Check sheet for the drawn part. Datum: minimum x, y, z corner. Units: mm. Round coordinates to 2 decimals unless told otherwise and drop trailing zeros. Write each loop counter-clockwise with the first axis right and the second up, starting at its lowest first coordinate (ties: lowest second). Pieces come first, ordered by that corner, then holes. Notation, with made-up numbers: (-40, 59) - (-34, 59) arc R13 ccw to (-34, 76) - close; hole circle Ø3 at (4.25, -29.5). An arc over 180 degrees is marked (long way). Answer as a JSON object with one key per item and string values. Group by question number.
1) Section check C-C (z = 4). Enter the section's corners in (x, y).
2) Section check B-B (y = 4). Enter the section's corners in (x, z), then the cut area to 3 significant figures.
3) Mould release check, pull along X, two halves, no side actions. Record for the marked faces 1, 2 and 3: +X half, -X half, draft (parallel to the pull), parting line (faces both ways), or undercut.
4) Thickness scan on line 1 (Z direction, x = 12.3, y = 2); line 2 (X direction, y = 4.5, z = 4.25); line 3 (Z direction, x = 13.25, y = 1.5). Record the ranges inside material, lowest first.
5) Section check D-D (x = 12.75). Enter the section's corners in (y, z).
6) Section check A-A (z = 5). Enter the section's corners in (x, y), then the cut area to 3 significant figures.
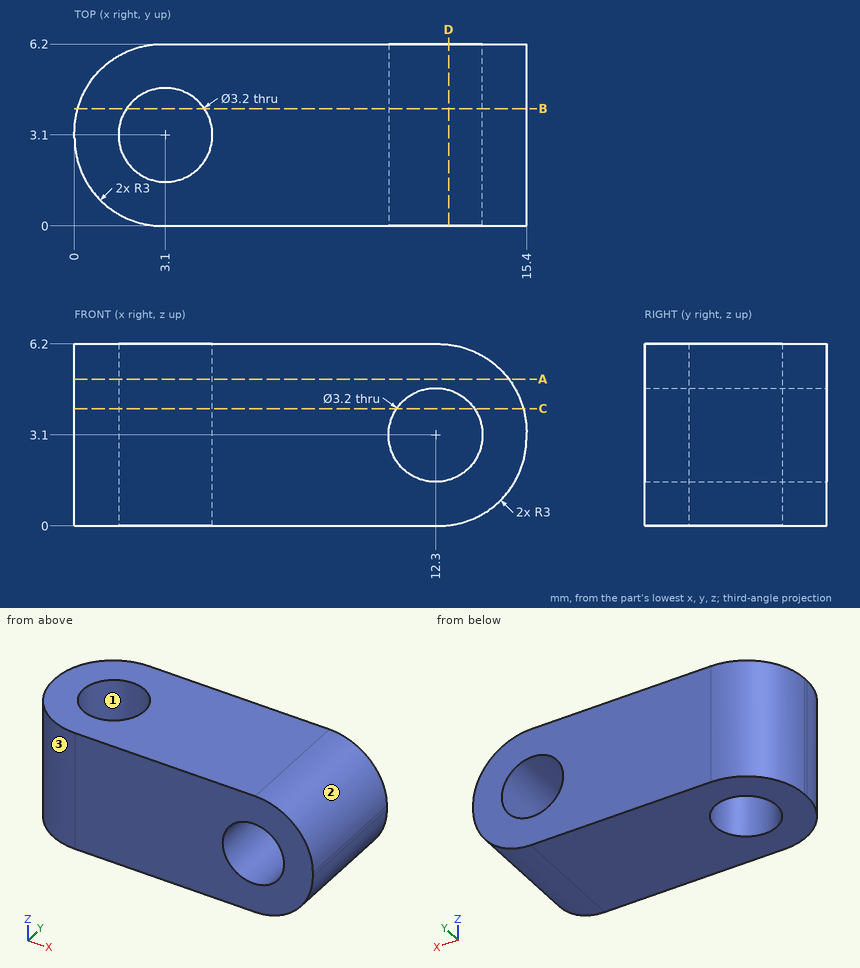
Returned:
{
 "1": {"outline": "(0, 3) arc R3 ccw to (3, 0) - (10.98, 0) - (10.98, 6.2) - (3, 6.2) arc R3 ccw to (0, 3.2) - close; (13.62, 0) - (15.29, 0) - (15.29, 6.2) - (13.62, 6.2) - close; hole circle Ø3.2 at (3.1, 3.1)"},
 "2": {"outline": "(0.11, 0) - (1.78, 0) - (1.78, 6.2) - (0.11, 6.2) - close; (4.42, 0) - (12.4, 0) arc R3 ccw to (15.4, 3) - (15.4, 3.2) arc R3 ccw to (12.4, 6.2) - (4.42, 6.2) - close; hole circle Ø3.2 at (12.3, 3.1)", "area": "66.5 mm2"},
 "3": {"face 1": "undercut", "face 2": "+X half", "face 3": "-X half"},
 "4": {"line 1": "0 to 1.5, 4.7 to 6.2", "line 2": "0.3 to 2.33, 3.87 to 11.19, 13.41 to 15.21", "line 3": "0.12 to 1.81, 4.39 to 6.08"},
 "5": {"outline": "(0, 0.02) - (6.2, 0.02) - (6.2, 1.56) - (0, 1.56) - close; (0, 4.64) - (6.2, 4.64) - (6.2, 6.18) - (0, 6.18) - close"},
 "6": {"outline": "(0, 3) arc R3 ccw to (3, 0) - (14.8, 0) - (14.8, 6.2) - (3, 6.2) arc R3 ccw to (0, 3.2) - close; hole circle Ø3.2 at (3.1, 3.1)", "area": "79.9 mm2"}
}
